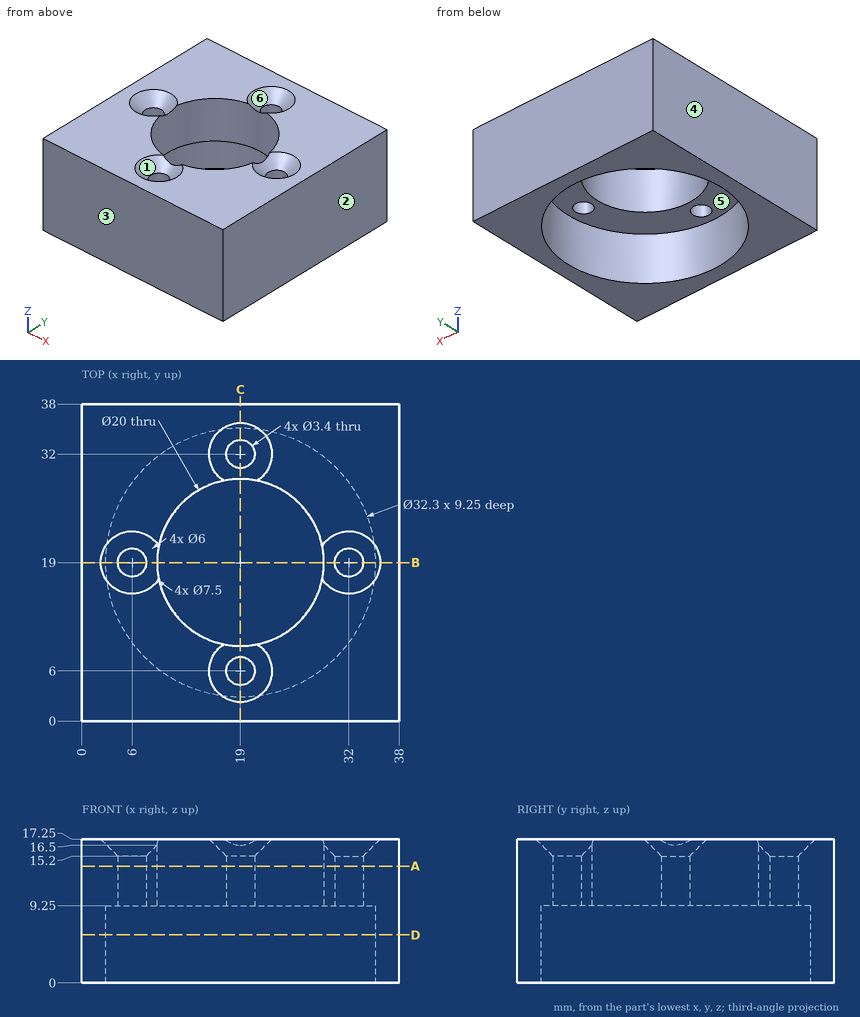
Answer from the drawing. Dimensions are ordinates in mm from the lowest x, y and z of the part. A direction names the side the tool comes from. Round coordinates to 2 decimals unless told otherwise and drop trailing zeros. Order: outer loops, then holes, each group sorted by start corner. A loop starts at its lowest first (then second) coordinate and runs counter-clockwise, first axis right, second up.
1) For the marked faces 5 and 6, determine the directions among +Z, -Z, +X, -X, +Y, -Y from which every point of the face is accessible in a straight line to the end or side of a thin tool.
2) Flat-ended cylindrical pins translate along their axes: pin 1 (1.5 mm diameter, centred on x = 23.5, y = 9, fed in from -Z); pin 2 (4 mm diameter, centred on x = 32, y = 19, fed in from +Z); pin 3 (9.5 mm diameter, centred on x = 17, y = 18.5, fed in from -Z). Find the tip coordinate at first contact, or state that the pin passes through.
3) The part is cut by section B-B on y = 19. Write down the section's boundary in (x, z), plus the area to 3 significant figures.
4) The part is cut by section A-A on z = 14. Write down the section's boundary in (x, y).
5) The part is cut by section D-D on z = 5.75. Write down the section's boundary in (x, y), plus the area to 3 significant figures.
6) Straight lines are drawn through the part: L1, parallel to Y at x = 19, z = 4.5; L2, parallel to X at y = 6, z = 11.85. For each, find the intervals that lie inside material, in ascending order.
7) The mould has two halves that part along X. Classify the marked faces 1, 2, 3 and 4: released by +X, released by -X, zero draft, split by the parting line, or undercut.
Resolved:
1. face 5: -Z
1. face 6: +Z
2. pin 1: stops at z = 9.25
2. pin 2: stops at z = 15.5
2. pin 3: passes through
3. outline: (0, 0) - (2.85, 0) - (2.85, 9.25) - (4.3, 9.25) - (4.3, 15.2) - (2.25, 17.25) - (0, 17.25) - close; (7.7, 9.25) - (9, 9.25) - (9, 16.5) - (7.7, 15.2) - close; (29, 9.25) - (30.3, 9.25) - (30.3, 15.2) - (29, 16.5) - close; (33.7, 9.25) - (35.15, 9.25) - (35.15, 0) - (38, 0) - (38, 17.25) - (35.75, 17.25) - (33.7, 15.2) - close
3. area: 134 mm2
4. outline: (0, 0) - (38, 0) - (38, 38) - (0, 38) - close; hole circle Ø3.4 at (6, 19); hole circle Ø20 at (19, 19); hole circle Ø3.4 at (19, 6); hole circle Ø3.4 at (19, 32); hole circle Ø3.4 at (32, 19)
5. outline: (0, 0) - (38, 0) - (38, 38) - (0, 38) - close; hole circle Ø32.3 at (19, 19)
5. area: 625 mm2
6. L1: y = 0 to 2.85, 35.15 to 38
6. L2: x = 0 to 17.3, 20.7 to 38
7. face 1: undercut
7. face 2: released by +X
7. face 3: zero draft
7. face 4: released by -X
